For this review, take the finished solid that the model builds, in its own axes (mm). Face numbers are marked on the shaded views. A direction names the side the tool comes from. Give positions to 0.01 mm unless a question says otherwise; leave off trailing zeros. Write each loop counter-clockwise with the first axis right and the second up, starting at its lowest first coordinate (ties: lowest second). Pieces come first, ordered by that corner, then holes. Notation, with made-up numbers: (31, -7) -> (43, -7) arc R32 cw to (43, 31) -> close; hole circle Ø7 at (-25.5, 52.25). An arc over 180 degrees is marked (long way). Return JSON: item names as keys, results as strings.
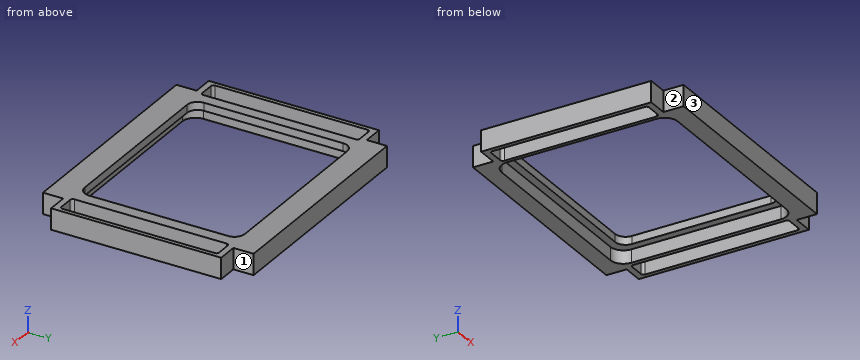
from build123d import *

# Parameters (mm, degrees)
BOSS_EXTRU_1_DEPTH      = 5
BOSS_EXTRU_2_DEPTH      = 3
ENL_V_MAT_EXTRU_9_DEPTH = 10
ENL_V_MAT_EXTRU_4_DEPTH = 9


with BuildPart() as part:
    # Esquisse1 → Boss.-Extru.1 (new body)
    with BuildSketch(Plane.XY):
        Polygon((-40.258600608, 39.883341456), (44.541399392, 39.883341456), (44.541399392, 32.183341456), (52.241399392, 32.183341456), (52.241399392, -32.616658544), (44.541399392, -32.616658544), (44.541399392, -40.316658544), (-40.258600608, -40.316658544), (-40.258600608, -32.616658544), (-47.958600608, -32.616658544), (-47.958600608, 32.183341456), (-40.258600608, 32.183341456), align=None)
        with BuildLine():
            Line((-32.483600608, 33.583341456), (36.516399392, 33.583341456))
            ThreePointArc((36.516399392, 33.583341456), (40.051933298, 32.118875362), (41.516399392, 28.583341456))
            Line((41.516399392, 28.583341456), (41.516399392, -28.416658544))
            ThreePointArc((41.516399392, -28.416658544), (40.051933298, -31.952192449), (36.516399392, -33.416658544))
            Line((36.516399392, -33.416658544), (-32.483600608, -33.416658544))
            ThreePointArc((-32.483600608, -33.416658544), (-36.019134514, -31.952192449), (-37.483600608, -28.416658544))
            Line((-37.483600608, -28.416658544), (-37.483600608, 28.583341456))
            ThreePointArc((-37.483600608, 28.583341456), (-36.019134514, 32.118875362), (-32.483600608, 33.583341456))
        make_face(mode=Mode.SUBTRACT)
    extrude(amount=BOSS_EXTRU_1_DEPTH)

    # Esquisse2 → Boss.-Extru.2 (add)
    with BuildSketch(Plane.XY.offset(5)):
        Polygon((-47.958600608, 32.183341456), (-40.258600608, 32.183341456), (-40.258600608, 39.883341456), (44.541399392, 39.883341456), (44.541399392, 32.183341456), (52.241399392, 32.183341456), (52.241399392, -32.616658544), (44.541399392, -32.616658544), (44.541399392, -40.316658544), (-40.258600608, -40.316658544), (-40.258600608, -32.616658544), (-47.958600608, -32.616658544), align=None)
    extrude(amount=BOSS_EXTRU_2_DEPTH)

    # Esquisse8 → Enlèv. mat.-Extru.9 (cut)
    with BuildSketch(Plane(origin=(0, 0, 5), x_dir=(-1, 0, 0), z_dir=(0, 0, -1))):
        with BuildLine():
            Line((-34.516399392, 30.583341456), (30.483600608, 30.583341456))
            ThreePointArc((30.483600608, 30.583341456), (33.312027733, 29.411768581), (34.483600608, 26.583341456))
            Line((34.483600608, 26.583341456), (34.483600608, -26.416658544))
            ThreePointArc((34.483600608, -26.416658544), (33.312027733, -29.245085668), (30.483600608, -30.416658544))
            Line((30.483600608, -30.416658544), (-34.516399392, -30.416658544))
            ThreePointArc((-34.516399392, -30.416658544), (-37.344826516, -29.245085668), (-38.516399392, -26.416658544))
            Line((-38.516399392, -26.416658544), (-38.516399392, 26.583341456))
            ThreePointArc((-38.516399392, 26.583341456), (-37.344826516, 29.411768581), (-34.516399392, 30.583341456))
        make_face()
    extrude(amount=-ENL_V_MAT_EXTRU_9_DEPTH, mode=Mode.SUBTRACT)

    # Esquisse6 → Enlèv. mat.-Extru.4 (cut, through all)
    with BuildSketch(Plane(origin=(0, 0, 0), x_dir=(-1, 0, 0), z_dir=(0, 0, -1))):
        with BuildLine():
            Line((-49.628899392, 29.783341456), (-44.128899392, 29.783341456))
            ThreePointArc((-44.128899392, 29.783341456), (-43.421792611, 29.490448238), (-43.128899392, 28.783341456))
            Line((-43.128899392, 28.783341456), (-43.128899392, -29.216658544))
            ThreePointArc((-43.128899392, -29.216658544), (-43.421792611, -29.923765325), (-44.128899392, -30.216658544))
            Line((-44.128899392, -30.216658544), (-49.628899392, -30.216658544))
            ThreePointArc((-49.628899392, -30.216658544), (-50.336006173, -29.923765325), (-50.628899392, -29.216658544))
            Line((-50.628899392, -29.216658544), (-50.628899392, 28.783341456))
            ThreePointArc((-50.628899392, 28.783341456), (-50.336006173, 29.490448238), (-49.628899392, 29.783341456))
        make_face()
        with BuildLine():
            Line((45.346100608, -30.216658544), (39.846100608, -30.216658544))
            ThreePointArc((39.846100608, -30.216658544), (39.138993827, -29.923765325), (38.846100608, -29.216658544))
            Line((38.846100608, -29.216658544), (38.846100608, 28.783341456))
            ThreePointArc((38.846100608, 28.783341456), (39.138993827, 29.490448238), (39.846100608, 29.783341456))
            Line((39.846100608, 29.783341456), (45.346100608, 29.783341456))
            ThreePointArc((45.346100608, 29.783341456), (46.053207389, 29.490448238), (46.346100608, 28.783341456))
            Line((46.346100608, 28.783341456), (46.346100608, -29.216658544))
            ThreePointArc((46.346100608, -29.216658544), (46.053207389, -29.923765325), (45.346100608, -30.216658544))
        make_face()
    extrude(amount=-ENL_V_MAT_EXTRU_4_DEPTH, mode=Mode.SUBTRACT)


solid = part.part
1. To check wall thickness, follow probe 1 along X at (y, z) = (20, 4); probe 2 along X at (y, z) = (22, 6.5); probe 3 along Y at (x, z) = (44.5, 6.75). State the ranges of each line that lie inside material, in increasing order.
Results found:
{"probe 1": "x = -47.96 to -46.35, -38.85 to -37.48, 41.52 to 43.13, 50.63 to 52.24", "probe 2": "x = -47.96 to -46.35, -38.85 to -34.48, 38.52 to 43.13, 50.63 to 52.24", "probe 3": "y = -40.32 to -30.22, 29.78 to 39.88"}
2. Add section C-C, the plane z = 6.75. Count the separate pieces of the cut face and the enclosed holes in it, plus the area to 3 significant figures.
Results found:
{"separate pieces": "1", "enclosed holes": "3", "area": "2,460 mm²"}
3. Add section B-B, the plane x = 3. State the section outline as (y, z) points, plus the area to 3 significant figures.
Results found:
{"outline": "(-40.32, 0) -> (-33.42, 0) -> (-33.42, 5) -> (-30.42, 5) -> (-30.42, 8) -> (-40.32, 8) -> close; (30.58, 5) -> (33.58, 5) -> (33.58, 0) -> (39.88, 0) -> (39.88, 8) -> (30.58, 8) -> close", "area": "124 mm²"}
4. Add section D-D, the plane y = -34.5. State the section outline as (x, z) points, plus the area to 3 significant figures.
Results found:
{"outline": "(-40.26, 0) -> (44.54, 0) -> (44.54, 8) -> (-40.26, 8) -> close", "area": "678 mm²"}
5. For pin 1 (4 mm diameter, centred on x = 49.5, z = 5, fed in from -Y); pin 2 (2.5 mm diameter, centred on y = -36.5, z = 4.5, fed in from +X), all flat-tipped, find the tip position at first contact; note any pin that passes through.
Results found:
{"pin 1": "stops at y = -32.62", "pin 2": "stops at x = 44.54"}
6. For the marked faces 1, 2 and 3, list the 3-axis set-ups (+Z, -Z, +X, -X, +Y, -Y) from which the entire face can be reached by the end or side of a thin tool; tool diameter is ignored.
Results found:
{"face 1": "+Z, -Z, +X, +Y", "face 2": "+Z, -Z, -X, -Y", "face 3": "+Z, -Z, +X, -X, -Y"}
7. Add section A-A, the plane y = 15. State the section outline as (x, z) points, plus the area to 3 significant figures.
Results found:
{"outline": "(-47.96, 0) -> (-46.35, 0) -> (-46.35, 8) -> (-47.96, 8) -> close; (-38.85, 0) -> (-37.48, 0) -> (-37.48, 5) -> (-34.48, 5) -> (-34.48, 8) -> (-38.85, 8) -> close; (38.52, 5) -> (41.52, 5) -> (41.52, 0) -> (43.13, 0) -> (43.13, 8) -> (38.52, 8) -> close; (50.63, 0) -> (52.24, 0) -> (52.24, 8) -> (50.63, 8) -> close", "area": "67.6 mm²"}
